The listing builds one solid part. Answer for the finished solid, in the listing's coordinates (mm). A direction names the side the tool comes from. Give positions to 0.01 mm unless a question says otherwise; leave off trailing zeros. Loops run counter-clockwise (first coordinate to the right, second up) from the corner with the lowest first, then second, coordinate; pieces in that order, holes last. Notation, with made-up numbers: M -12,51 L 4,51 A35 ccw 4,87 Z; hole C 37.5,29 d8. An arc over 180 degrees is marked long. Return JSON: item names as keys, results as strings.
from build123d import *

# Parameters (mm, degrees)
SKETCH3_W           = 134
SKETCH3_H           = 104
SKETCH3_W_2         = 94
SKETCH3_H_2         = 64
BOSS_EXTRUDE2_DEPTH = 35
SKETCH3_6_W         = 94
SKETCH3_6_H         = 64
BOSS_EXTRUDE3_DEPTH = 5
SKETCH8_W           = 134
SKETCH8_H           = 104
SKETCH8_W_2         = 104
SKETCH8_H_2         = 74
CUT_EXTRUDE3_DEPTH  = 30
CUT_EXTRUDE4_DEPTH  = 114
SKETCH9_W           = 94
SKETCH9_H           = 10
CUT_EXTRUDE5_DEPTH  = 5
SKETCH10_W          = 17
SKETCH10_H          = 10
CUT_EXTRUDE6_DEPTH  = 5
SKETCH11_W          = 28.983298244
SKETCH11_H          = 12.432282013
BOSS_EXTRUDE4_DEPTH = 5
SKETCH13_W          = 12
SKETCH13_H          = 6
CUT_EXTRUDE7_DEPTH  = 10


with BuildPart() as part:
    # Sketch3 → Boss-Extrude2 (new body)
    with BuildSketch(Plane(origin=(0, 0, 0), x_dir=(1, 0, 0), z_dir=(0, 1, 0))):
        Rectangle(SKETCH3_W, SKETCH3_H)
        Rectangle(SKETCH3_W_2, SKETCH3_H_2, mode=Mode.SUBTRACT)
    extrude(amount=BOSS_EXTRUDE2_DEPTH)

    # Sketch3<6> → Boss-Extrude3 (add)
    with BuildSketch(Plane(origin=(0, 0, 0), x_dir=(1, 0, 0), z_dir=(0, 1, 0))):
        Rectangle(SKETCH3_6_W, SKETCH3_6_H)
    extrude(amount=BOSS_EXTRUDE3_DEPTH)

    # Sketch8 → Cut-Extrude3 (cut)
    with BuildSketch(Plane(origin=(0, 35, 0), x_dir=(1, 0, 0), z_dir=(0, 1, 0))):
        Rectangle(SKETCH8_W, SKETCH8_H)
        Rectangle(SKETCH8_W_2, SKETCH8_H_2, mode=Mode.SUBTRACT)
    extrude(amount=-CUT_EXTRUDE3_DEPTH, mode=Mode.SUBTRACT)

    # Sketch5 → Cut-Extrude4 (cut)
    with BuildSketch(Plane(origin=(67, 0, 0), x_dir=(0, 0, -1), z_dir=(1, 0, 0))):
        Polygon((32, 5.263033051), (32, 24), (-13, 24), (-13, 5), (32, 5), align=None)
    extrude(amount=-CUT_EXTRUDE4_DEPTH, mode=Mode.SUBTRACT)

    # Sketch9 → Cut-Extrude5 (cut)
    with BuildSketch(Plane.XY.offset(37)):
        with Locations((0, 10)):
            Rectangle(SKETCH9_W, SKETCH9_H)
    extrude(amount=-CUT_EXTRUDE5_DEPTH, mode=Mode.SUBTRACT)

    # Sketch10 → Cut-Extrude6 (cut)
    with BuildSketch(Plane(origin=(0, 0, -37), x_dir=(-1, 0, 0), z_dir=(0, 0, -1))):
        with Locations((-38.5, 10)):
            Rectangle(SKETCH10_W, SKETCH10_H)
    extrude(amount=-CUT_EXTRUDE6_DEPTH, mode=Mode.SUBTRACT)

    # Sketch11 → Boss-Extrude4 (add)
    with BuildSketch(Plane(origin=(0, 0, -37), x_dir=(-1, 0, 0), z_dir=(0, 0, -1))):
        with Locations((-34.333019182, 11.216141007)):
            Rectangle(SKETCH11_W, SKETCH11_H)
    extrude(amount=-BOSS_EXTRUDE4_DEPTH)

    # Sketch13 → Cut-Extrude7 (cut)
    with BuildSketch(Plane(origin=(0, 0, -37), x_dir=(-1, 0, 0), z_dir=(0, 0, -1))):
        with Locations((-33, 8)):
            Rectangle(SKETCH13_W, SKETCH13_H)
    extrude(amount=-CUT_EXTRUDE7_DEPTH, mode=Mode.SUBTRACT)


solid = part.part
(1) Given pin 1 (9 mm diameter, centred on y = 22.5, z = 1, fed in from -X); pin 2 (15 mm diameter, centred on y = 25.5, z = 0.5, fed in from +X); pin 3 (1.5 mm diameter, centred on x = 13.5, y = 15.5, fed in from -Z); pin 4 (5.5 mm diameter, centred on x = 49.5, z = 1, fed in from -Y), each flat-ended and moving along its own axis, determine where each tip first touches the part or whether it passes through.
Values follow:
{"pin 1": "x = -52", "pin 2": "x = 52", "pin 3": "z = -37", "pin 4": "y = 0"}
(2) Straight lines are drawn through the part: line 1 along Z through (x, y) = (18.5, 25.5); line 2 along Z through (x, y) = (50, 11.5); line 3 along Y through (x, z) = (38, -5.5). For each, find the intervals that lie inside material, in ascending order.
Values follow:
{"line 1": "-37 to -32, 32 to 37", "line 2": "-37 to -32, 13 to 37", "line 3": "0 to 5"}
(3) A tool of negligible diameter and unlimited length cuts with its end or side. For faces 5 (the flat face through (-1, 20, -37)), 6 (the flat face through (-1, 15, 35)), 7 (the flat face through (50, 15, 13)), 8 (the flat face through (27, 8, -35)), 9 (the flat face through (-52, 20, 1)), from which of +Z, -Z, +X, -X, +Y, -Y can it reach the whole face along a straight path? Write none if from no direction.
Values follow:
{"face 5": "-Z, +X, -X, +Y", "face 6": "+Z", "face 7": "+X", "face 8": "+Z, -Z", "face 9": "+Z, -Z, -X, +Y"}
(4) The part is cut by section A-A (x = 16). Determine the outline of the cut face in (y, z), and give its area (3 significant figures).
Values follow:
{"outline": "M 0,-52 L 5,-52 L 5,-37 L 35,-37 L 35,-32 L 5,-32 L 5,52 L 0,52 Z; M 15,32 L 35,32 L 35,37 L 15,37 Z", "area": "770 mm²"}
(5) The part is cut by section B-B (z = 8). Determine the outline of the cut face in (x, y), and give its area (3 significant figures).
Values follow:
{"outline": "M -67,0 L 67,0 L 67,5 L -47,5 L -47,35 L -52,35 L -52,5 L -67,5 Z; M 47,24 L 52,24 L 52,35 L 47,35 Z", "area": "875 mm²"}
(6) The part is cut by section D-D (y = 29). Determine the outline of the cut face in (x, z).
Values follow:
{"outline": "M -52,-37 L 52,-37 L 52,37 L -52,37 Z; hole M -47,-32 L 47,-32 L 47,32 L -47,32 Z"}
(7) Determine the mould class of faces 1 (the flat face through (67, 2, 1)), 2 (the flat face through (-4, 35, 33)), 3 (the flat face through (33, 11, -35)), 4 (the flat face through (50, 24, -10)) for opening direction Y: released by +Y, released by -Y, zero draft, split by the parting line, or undercut.
Values follow:
{"face 1": "zero draft", "face 2": "released by +Y", "face 3": "undercut", "face 4": "undercut"}
(8) The part is cut by section C-C (y = 9). Determine the outline of the cut face in (x, z).
Values follow:
{"outline": "M -52,-37 L 27,-37 L 27,-32 L -47,-32 L -47,37 L -52,37 Z; M 39,-37 L 52,-37 L 52,-32 L 39,-32 Z; M 47,13 L 52,13 L 52,37 L 47,37 Z"}
